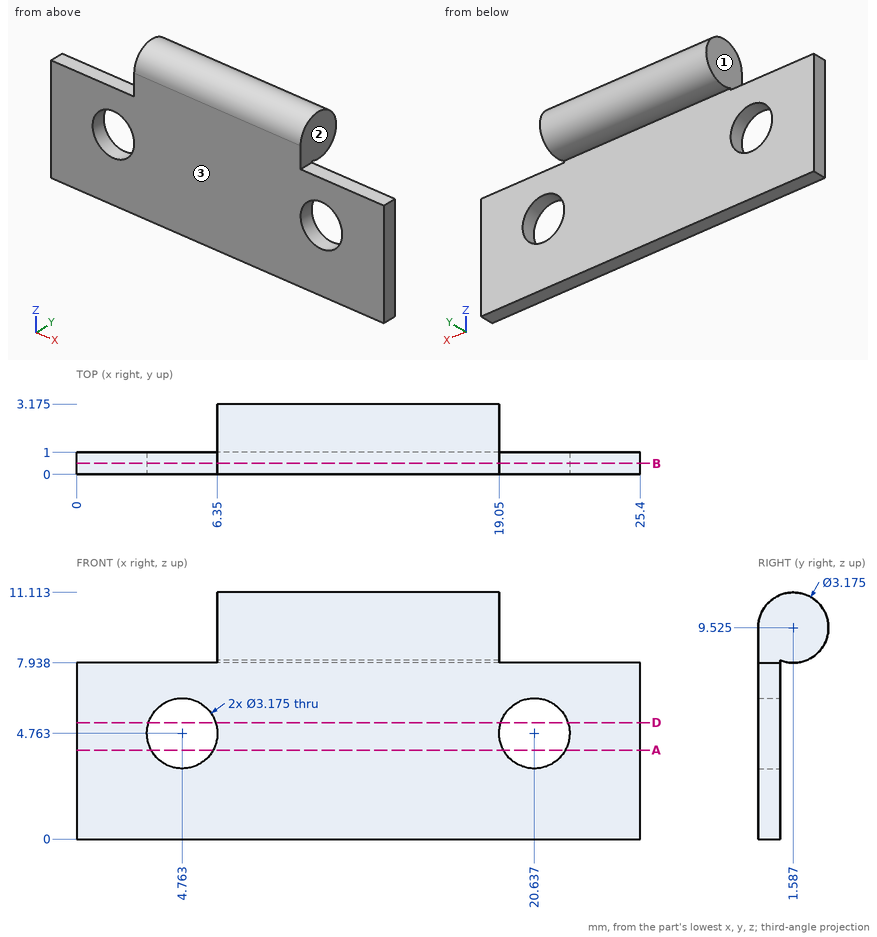
The drawing under review shows one solid part. Ordinate dimensions are in mm from its lowest x, y, z. A direction names the side the tool comes from. Round coordinates to 2 decimals unless told otherwise and drop trailing zeros. Order: outer loops, then holes, each group sorted by start corner. A loop starts at its lowest first (then second) coordinate and runs counter-clockwise, first axis right, second up. Notation, with made-up numbers: (-29, 34.25) -> (-9, 34.25) arc R21 cw to (-9, 46.25) -> close; hole circle Ø7 at (63.5, 16.5). An arc over 180 degrees is marked (long way). Use a Markdown table: item, result.
Q1. We need section B-B on y = 0.5. State how many separate pieces and enclosed holes the cut face has, then the cut area to 3 significant figures.
Values:
| item | result |
|---|---|
| separate pieces | 1 |
| enclosed holes | 2 |
| area | 221 mm^2 |
Q2. We need section D-D on z = 5.25. Write out the cut boundary in (x, y).
Values:
| item | result |
|---|---|
| outline | (0, 0) -> (3.25, 0) -> (3.25, 1) -> (0, 1) -> close; (6.27, 0) -> (19.13, 0) -> (19.13, 1) -> (6.27, 1) -> close; (22.15, 0) -> (25.4, 0) -> (25.4, 1) -> (22.15, 1) -> close |
Q3. Clearance check with flat-ended pins moving along their axes: P1, Ø4, axis at x = 13.5, z = 2.5, coming from the +Y side; P2, Ø1.6, axis at y = 1.5, z = 9, coming from the +X side. State where each tip first meets the part, or that it passes through.
Values:
| item | result |
|---|---|
| P1 | stops at y = 1 |
| P2 | stops at x = 19.05 |
Q4. Tool access review of the marked faces 1, 2 and 3: name each direction out of +Z, -Z, +X, -X, +Y, -Y from which nothing blocks a thin tool from reaching the whole face with its end or side.
Values:
| item | result |
|---|---|
| face 1 | +Z, -X, +Y, -Y |
| face 2 | +Z, +X, +Y, -Y |
| face 3 | +Z, -Z, +X, -X, -Y |
Q5. For line 1 (X direction, y = 2.8, z = 10); line 2 (Z direction, x = 23, y = 0.4); line 3 (Y direction, x = 2.5, z = 1), list the stretches that pass through material, from the lowest coordinate up.
Values:
| item | result |
|---|---|
| line 1 | x = 6.35 to 19.05 |
| line 2 | z = 0 to 7.94 |
| line 3 | y = 0 to 1 |
Q6. We need section A-A on z = 4. Write out the cut boundary in (x, y) (1 decimal).
Values:
| item | result |
|---|---|
| outline | (0, 0) -> (3.4, 0) -> (3.4, 1) -> (0, 1) -> close; (6.2, 0) -> (19.2, 0) -> (19.2, 1) -> (6.2, 1) -> close; (22, 0) -> (25.4, 0) -> (25.4, 1) -> (22, 1) -> close |
